Read the model definition and answer for the solid it produces. Units are mm, in the model's axes. A direction names the side the tool comes from. Give positions to 0.01 mm unless a question says otherwise; leave off trailing zeros. Order: outer loops, then holes, each group sorted by start corner. A loop starts at its lowest first (then second) coordinate and runs counter-clockwise, first axis right, second up. Notation, with made-up numbers: (29.5, -32) - (56.5, -32) arc R27 ccw to (56.5, 5) - close; hole circle Ø7 at (79.25, 24.25). An arc over 180 degrees is marked (long way). Write each question's results on one line, items separated by ' | '. Start each with the question number.
Q1. For a pull along Y with two mould halves and no side action, classify faces 1 (the face through (-0.2, 2.5, 12.2)), 2 (the face through (0.867, 0.986, 3.905)), 3 (the face through (0, 2, -5)) as +Y half, -Y half, draft (parallel to the pull), parting line (faces both ways), or undercut.
Q2. Find section C-C on y = 71.5. Give the vertices of the cut face in (x, z).
Q3. Find the intervals of material crossed by line 1 along Z through (x, y) = (0, 0.6); line 2 along X through (y, z) = (63, 0); line 3 along Y through (x, z) = (-6, 3.5), in increasing order. Write a range as from..to.
Q4. Find section D-D on y = 41. Give the vertices of the cut face in (x, z).
Q5. Find section A-A on y = 23. Give the vertices of the cut face in (x, z).
Q6. Flat-ended cylindrical pins translate along their axes: P1, Ø7.5, axis at y = 26.5, z = -9, coming from the +X side; P2, Ø2, axis at y = 27.5, z = -6.5, coming from the -X side; P3, Ø6, axis at x = 8, y = 39.5, coming from the +Z side; P4, Ø1.6, axis at x = 0, z = 8, coming from the +Y side. Find the tip coordinate at first contact, or state that the pin passes through.
Q7. A tool of negligible diameter and unlimited length cuts with its end or side. For faces 4 (the face through (13, 94, 0)), 5 (the face through (0.2, 47.5, -12)), 6 (the face through (10.161, 54.558, -4.213)), from which of +Z, -Z, +X, -X, +Y, -Y can it reach the whole face along a straight path? Write none if from no direction.
Autodesk Inventor part; units mm, degrees
ref_plane "YZ Plane" through (0, 0, 0) normal (1, 0, 0) x (0, 1, 0)
ref_plane "XZ Plane" through (0, 0, 0) normal (0, 1, 0) x (-1, 0, 0)
ref_plane "XY Plane" through (0, 0, 0) normal (0, 0, 1) x (1, 0, 0)
sketch "Sketch1" plane through (0, 0, 0) normal (0, 1, 0) x (-1, 0, 0)
  circle A0 centre (0, 0) radius 4
  circle A1 centre (0, 0) radius 15
  circle A2 centre (0, -8) radius 1
  circle A3 centre (0, 8) radius 1
  dimension "d0" = 30
  dimension "d1" = 8
  dimension "d2" = 8
  dimension "d3" = 2
  dimension "d4" = 2
  dimension "d5" = 8
extrude "Extrusion1" add sketch "Sketch1" along normal blind 2
sketch "Sketch2" plane through (0, 2, 0) normal (0, 1, 0) x (1, 0, 0)
  circle A0 centre (0, 0) radius 15
  line L0 (0, 0) -> (18.7194, 0) construction
  circle A1 centre (0, 0) radius 11
  dimension "d33" = 22
extrude "Extrusion2" add sketch "Sketch2" along normal blind 87
sketch "Sketch3" plane through (0, 89, 0) normal (0, 1, 0) x (1, 0, 0)
  circle A0 centre (13, 0) radius 2
  circle A1 centre (-13, 0) radius 2
  point P0 (0, 0)
  dimension "d15" = 4
  dimension "d16" = 4
  dimension "d17" = 13
  dimension "d18" = 13
extrude "Extrusion3" add sketch "Sketch3" along normal blind 5
sketch "Sketch4" plane through (0, 2, 0) normal (0, 1, 0) x (1, 0, 0)
  circle A0 centre (0, -8) radius 1
  circle A1 centre (0, 8) radius 1
  point P0 (0, 0)
hole "Hole1" at (0, 2, 8) at (0, 2, -8) direction (0, -1, 0) diameter 1.567 depth 2 countersink diameter 4 countersink angle 90
sketch "Sketch6" plane through (0, 0, 0) normal (0, 0, 1) x (1, 0, 0)
  line L0 (0, 37.5) -> (0, 12.5) construction
  line L1 (-10, 37.5) -> (-10, 12.5)
  line L2 (10, 12.5) -> (10, 37.5)
  arc A0 (10, 37.5) -> (-10, 37.5) centre (0, 37.5) ccw
  arc A1 (-10, 12.5) -> (10, 12.5) centre (0, 12.5) ccw
  line L3 (-4, 2) -> (4, 2)
  point P0 (0, 0)
  point P1 (0, 25)
  point P2 (-3.1225, 2)
  point P3 (3.1225, 2)
  dimension "d28" = 20
  dimension "d29" = 25
  dimension "d30" = 23
extrude "Extrusion4" cut sketch "Sketch6" against normal mid plane 40
properties part number "Lock"
Working result:
1) face 1: undercut | face 2: draft | face 3: +Y half
2) outline: circle Ø30 at (0, 0); hole circle Ø22 at (0, 0)
3) line 1: -15..-9, -7..-4, 4..7, 9..15 | line 2: -15..-11, 11..15 | line 3: 0..2
4) outline: (-9.37, -11.72) - (-9.37, -5.77) arc R11 cw to (-9.37, 5.77) - (-9.37, 11.72) arc R15 ccw to start; (9.37, -11.72) arc R15 ccw to (9.37, 11.72) - (9.37, 5.77) arc R11 cw to (9.37, -5.77) - close
5) outline: (-10, -11.18) - (-10, -4.58) arc R11 cw to (-10, 4.58) - (-10, 11.18) arc R15 ccw to start; (10, -11.18) arc R15 ccw to (10, 11.18) - (10, 4.58) arc R11 cw to (10, -4.58) - close
6) P1: x = 14.05 | P2: x = -13.96 | P3: z = 12.21 | P4: through
7) face 4: +Z, -Z, +X, -X, +Y | face 5: +Z, -Z | face 6: +Y
